from build123d import *

# Parameters (mm, degrees)
F0_R     = 4.2
F1_DEPTH = 5
F3_DEPTH = 5


# Not quite as in the source:
# - a pattern or mirror of a feature is missing from the dataset's text; its kind, count and spacing are read off the source's solid


with BuildPart() as f1:
    # F0 (on Front) → F1 (new body)
    with BuildSketch(Plane.XZ):
        with BuildLine():
            Line((-6, 20), (-6, 0))
            ThreePointArc((-6, 0), (0, -6), (6, 0))
            Line((6, 0), (6, 20))
            ThreePointArc((6, 20), (0, 26), (-6, 20))
        make_face()
        Circle(F0_R, mode=Mode.SUBTRACT)
        with Locations((0, 20)):
            Circle(F0_R, mode=Mode.SUBTRACT)
    extrude(amount=F1_DEPTH)

    # F2 (on face) → F3 (join, through all)
    with BuildSketch(Plane.XZ.offset(5)):
        Polygon((-0.85, 16.5869111364), (-0.85, 15.8869111364), (0, 14.8420017213), (0.85, 15.8869111364), (0.85, 16.5869111364), align=None)
    f3 = extrude(amount=-F3_DEPTH)

    # F3_copies: F3 across plane
    add(f3.mirror(Plane(origin=(0, 0, 10), x_dir=(-1, 0, 0), z_dir=(0, 0, -1))))


solid = f1.part
Can you work these out from the model? Positions are in its coordinate system, mm. A direction names the side the tool comes from. Coordinates: 2 decimals unless noted, no trailing zeros. Loops run counter-clockwise (first coordinate to the right, second up) from the corner with the lowest first, then second, coordinate; pieces in that order, holes last. Notation, with made-up numbers: M 20.25,-40 L 59.25,-40 A19 ccw 59.25,-15 Z; hole C 29.25,55.25 d8. An arc over 180 degrees is marked long. Return JSON: item names as keys, results as strings. Group by question number.
Item 1: Imagine slicing it at D-D (x = 3.75). Please give me the cut outline in (y, z).
Item 2: Imagine slicing it at B-B (y = -3.85). Please give me the cut outline in (x, z).
Item 3: Imagine slicing it at A-A (x = 0). Please give me the cut outline in (y, z), and give its area (3 significant figures).
Item 4: On a 3-axis mill with a long thin cutter (end or side, diameter ignored), from which of +Z, -Z, +X, -X, +Y, -Y can I reach the whole of each face in a straight line? I mean faces 5 (the flat face through (0, -5, 10)), 6 (the flat face through (0, -3, 3.413)). Say none if no direction works.
Item 5: I'm going to push flat-ended pins straight in: pin 1 Ø3 at (y, z) = (-3.5, 22.5) entering from +X; pin 2 Ø1 at (y, z) = (-2, 22.5) entering from -X. Where does each tip first touch, or does it pass through?
Item 6: If I drill on L1, parallel to Z at x = 0, y = -2.5; L2, parallel to Z at x = -2.5, y = -4.25; L3, parallel to X at y = -1.4, z = 20, over which ranges is the centre line in solid material (lowest first)? Write a range as from..to.
Item 7: Imagine slicing it at C-C (z = 23.5). Please give me the cut outline in (x, y).
Item 8: Thinking about a two-plate mould opening in Z: for faces 1 (the cylindrical face through (-0.173, -2.465, -4.196)), 2 (the flat face through (0, -3, 16.587)), 3 (the cylindrical face through (0, -2, 26)), 4 (the flat face through (0, 0, 10)), which applies, released by +Z, released by -Z, zero draft, split by the parting line, or undercut?
Verdict:
{
 "1": {"outline": "M -5,-4.68 L 0,-4.68 L 0,-1.89 L -5,-1.89 Z; M -5,1.89 L 0,1.89 L 0,18.11 L -5,18.11 Z; M -5,21.89 L 0,21.89 L 0,24.68 L -5,24.68 Z"},
 "2": {"outline": "M -6,0 A6 ccw 6,0 L 6,20 A6 ccw -6,20 Z; hole M -0.85,3.41 L -0.85,4.11 A4.2 ccw long 0.85,4.11 L 0.85,3.41 Z; hole M -0.85,15.89 L -0.85,16.59 L 0.85,16.59 L 0.85,15.89 A4.2 ccw long Z"},
 "3": {"outline": "M -5,-6 L 0,-6 L 0,-4.2 L -5,-4.2 Z; M -5,3.41 L 0,3.41 L 0,16.59 L -5,16.59 Z; M -5,24.2 L 0,24.2 L 0,26 L -5,26 Z", "area": "83.9 mm^2"},
 "4": {"face 5": "+Z, -Z, +X, -X, -Y", "face 6": "+Y, -Y"},
 "5": {"pin 1": "stops at x = 5.92", "pin 2": "stops at x = -5.66"},
 "6": {"L1": "z = -6..-4.2, 3.41..16.59, 24.2..26", "L2": "z = -5.45..-3.37, 3.37..16.63, 23.37..25.45", "L3": "x = -6..-4.2, 4.2..6"},
 "7": {"outline": "M -4.87,-5 L -2.32,-5 L -2.32,0 L -4.87,0 Z; M 2.32,-5 L 4.87,-5 L 4.87,0 L 2.32,0 Z"},
 "8": {"face 1": "undercut", "face 2": "undercut", "face 3": "released by +Z", "face 4": "zero draft"}
}
